from build123d import *

# Parameters (mm, degrees)
BOSS_EXTRUDE1_DEPTH       = 150
CUT_EXTRUDE1_REACH        = 34
SKETCH2_R                 = 12.5
CUT_EXTRUDE2_REACH        = 34
SKETCH3_R                 = 2.1
F_3_0MM_DOWEL_HOLE1_D     = 3
F_3_0MM_DOWEL_HOLE1_DEPTH = 2
F_3_0MM_DOWEL_HOLE2_D     = 3
F_3_0MM_DOWEL_HOLE2_DEPTH = 2.001


with BuildPart() as part:
    # Sketch1 → Boss-Extrude1 (new body)
    with BuildSketch(Plane.XY):
        Polygon((-75, 16), (75, 16), (75, -14), (105, -14), (105, -16), (73, -16), (73, 14), (-73, 14), (-73, -16), (-105, -16), (-105, -14), (-75, -14), align=None)
    extrude(amount=-BOSS_EXTRUDE1_DEPTH)

    # Sketch2 → Cut-Extrude1 (cut, up to next)
    with BuildSketch(Plane(origin=(0, 16, 0), x_dir=(1, 0, 0), z_dir=(0, 1, 0)), mode=Mode.PRIVATE) as cut_extrude1_sk1:
        with Locations((0, 67)):
            Circle(SKETCH2_R)
    cut_extrude1_tool1 = extrude(cut_extrude1_sk1.sketch, amount=-CUT_EXTRUDE1_REACH, mode=Mode.PRIVATE) & part.part
    add(cut_extrude1_tool1.solids().sort_by_distance((0, 16, -67))[0], mode=Mode.SUBTRACT)

    # Sketch3 → Cut-Extrude2 (cut, up to next)
    with BuildSketch(Plane(origin=(0, 16, 0), x_dir=(1, 0, 0), z_dir=(0, 1, 0)), mode=Mode.PRIVATE) as cut_extrude2_sk1:
        with Locations((17.5, 67)):
            Circle(SKETCH3_R)
    cut_extrude2_tool1 = extrude(cut_extrude2_sk1.sketch, amount=-CUT_EXTRUDE2_REACH, mode=Mode.PRIVATE) & part.part
    add(cut_extrude2_tool1.solids().sort_by_distance((17.5, 16, -67))[0], mode=Mode.SUBTRACT)
    # Sketch3 → Cut-Extrude2 (cut, up to next)
    with BuildSketch(Plane(origin=(0, 16, 0), x_dir=(1, 0, 0), z_dir=(0, 1, 0)), mode=Mode.PRIVATE) as cut_extrude2_sk2:
        with Locations((-17.5, 67)):
            Circle(SKETCH3_R)
    cut_extrude2_tool2 = extrude(cut_extrude2_sk2.sketch, amount=-CUT_EXTRUDE2_REACH, mode=Mode.PRIVATE) & part.part
    add(cut_extrude2_tool2.solids().sort_by_distance((-17.5, 16, -67))[0], mode=Mode.SUBTRACT)

    # Ø3.0mm Dowel Hole1
    with Locations(Plane(origin=(0, 14, 0), x_dir=(-1, 0, 0), z_dir=(0, -1, 0))):
        with Locations((56.5, 97.5), (56.5, 112.5), (56.5, 52.5), (56.5, 37.5), (36.5, 16.5), (21.5, 16.5), (-21.5, 16.5), (-36.5, 16.5), (-56.5, 37.5), (-56.5, 52.5), (-56.5, 97.5), (-56.5, 112.5), (-36.5, 133.5), (-21.5, 133.5), (36.5, 133.5), (21.5, 133.5)):
            Hole(F_3_0MM_DOWEL_HOLE1_D / 2, depth=F_3_0MM_DOWEL_HOLE1_DEPTH)

    # Ø3.0mm Dowel Hole2
    with Locations(Plane.ZY.offset(-73)):
        with Locations((-112.5, -2.5), (-97.5, -2.5), (-52.5, -2.5), (-37.5, -2.5)):
            f_3_0mm_dowel_hole2 = Hole(F_3_0MM_DOWEL_HOLE2_D / 2, depth=F_3_0MM_DOWEL_HOLE2_DEPTH)

    # Mirror1: Ø3.0mm Dowel Hole2 across plane
    add(f_3_0mm_dowel_hole2.mirror(Plane(origin=(0, 0, 0), x_dir=(0, 0, 1), z_dir=(1, 0, 0))), mode=Mode.SUBTRACT)


solid = part.part
Can you work these out from the model? Positions are in its coordinate system, mm. A direction names the side the tool comes from. Give positions to 0.01 mm unless a question says otherwise; leave off trailing zeros. Loops run counter-clockwise (first coordinate to the right, second up) from the corner with the lowest first, then second, coordinate; pieces in that order, holes last. Notation, with made-up numbers: (86, 15) -> (110, 15) arc R17 cw to (110, 20) -> close; hole circle Ø11 at (-14, 4). An arc over 180 degrees is marked (long way). Return JSON: item names as keys, results as strings.
Q1. I need wall thicknesses on probe 1 along Z at (x, y) = (-21.5, 15.45); probe 2 along X at (y, z) = (15.5, -133.5); probe 3 along X at (y, z) = (-13, -131.5). Which ranges of each line are inside material? Lowest first, please.
Checks:
{"probe 1": "z = -150 to -135, -132 to -18, -15 to 0", "probe 2": "x = -75 to -38, -35 to -23, -20 to 20, 23 to 35, 38 to 75", "probe 3": "x = -75 to -73, 73 to 75"}
Q2. I want a section at C-C, the plane z = -59. List the corners of the cut face in (x, y) for me.
Checks:
{"outline": "(-105, -16) -> (-73, -16) -> (-73, 14) -> (-9.6, 14) -> (-9.6, 16) -> (-75, 16) -> (-75, -14) -> (-105, -14) -> close; (9.6, 14) -> (73, 14) -> (73, -16) -> (105, -16) -> (105, -14) -> (75, -14) -> (75, 16) -> (9.6, 16) -> close"}
Q3. I want a section at A-A, the plane y = 3. List the corners of the cut face in (x, z) for me.
Checks:
{"outline": "(-75, -150) -> (-73, -150) -> (-73, 0) -> (-75, 0) -> close; (73, -150) -> (75, -150) -> (75, 0) -> (73, 0) -> close"}
Q4. I want a section at D-D, the plane z = -26. List the corners of the cut face in (x, y) for me.
Checks:
{"outline": "(-105, -16) -> (-73, -16) -> (-73, 14) -> (73, 14) -> (73, -16) -> (105, -16) -> (105, -14) -> (75, -14) -> (75, 16) -> (-75, 16) -> (-75, -14) -> (-105, -14) -> close"}
Q5. I want a section at B-B, the plane x = 17.5. List the corners of the cut face in (y, z) for me, then the cut area to 3 significant figures.
Checks:
{"outline": "(14, -150) -> (16, -150) -> (16, -69.1) -> (14, -69.1) -> close; (14, -64.9) -> (16, -64.9) -> (16, 0) -> (14, 0) -> close", "area": "292 mm2"}
Q6. On a 3-axis mill with a long thin cutter (end or side, diameter ignored), from which of +Z, -Z, +X, -X, +Y, -Y can I reach the whole of each face in a straight line? I mean faces 4 (the face through (75, 1, -74)), 5 (the face through (0.5, 14.3, -150)), 6 (the face through (-73, -1, -74)), 7 (the face through (-90, -14, -74)), 8 (the face through (-89, -16, -74)). Say none if no direction works.
Checks:
{"face 4": "+Z, -Z, +X, +Y", "face 5": "-Z, +X, -X, +Y, -Y", "face 6": "+Z, -Z, -Y", "face 7": "+Z, -Z, -X, +Y", "face 8": "+Z, -Z, +X, -X, -Y"}
Q7. We'd pull the mould along X, two halves only. Please class faces 1 (the face through (-15, 14, -74)), 2 (the face through (-75, 1, -74)), 3 (the face through (90, -14, -74)): released by +X, released by -X, zero draft, split by the parting line, or undercut.
Checks:
{"face 1": "undercut", "face 2": "released by -X", "face 3": "zero draft"}
Q8. For pin 1 Ø15 at (y, z) = (-1, -85.5) entering from +X; pin 2 Ø10 at (x, z) = (42, -90) entering from -Y; pin 3 Ø5 at (x, z) = (56.5, -52.5) entering from +Y; pin 4 Ø15 at (x, z) = (95.5, -68) entering from +Y, each with a flat end and sliding along its axis, tell me the tip position at first contact or that it passes through.
Checks:
{"pin 1": "stops at x = 75", "pin 2": "stops at y = 14", "pin 3": "stops at y = 16", "pin 4": "stops at y = -14"}
